For this review, take the finished solid that the model builds, in its own axes (mm). Round coordinates to 2 decimals unless told otherwise and drop trailing zeros. Write each loop counter-clockwise with the first axis right and the second up, starting at its lowest first coordinate (ties: lowest second). Pieces come first, ordered by that corner, then holes. Notation, with made-up numbers: (-37.75, -12) -> (-25.75, -12) arc R8 ccw to (-25.75, 3) -> close; hole circle Ø2 at (51, 53.25). An arc over 180 degrees is marked (long way). Answer as CSV lines item,"result". Start each with the question number.
Item 1: For pin 1 Ø8 at (x, y) = (50, 0) entering from +Z, flat-tipped, find the tip position at first contact; note if it passes through.
Item 2: Take a section at A-A on x = 50. Give the boundary of the cut face in (y, z), then the cut area to 3 significant figures.
Item 3: Take a section at B-B on y = 0. Give the boundary of the cut face in (x, z), then the cut area to 3 significant figures.
Item 4: Take a section at D-D on y = 4.75. Give the boundary of the cut face in (x, z), then the cut area to 3 significant figures.
Item 5: Take a section at C-C on z = 0.45. Give the boundary of the cut face in (x, y).
Item 6: Wall thickness on probe 1 along Y at (x, z) = (-50, -0.65); probe 2 along X at (y, z) = (3.5, 0.75); probe 3 along X at (y, z) = (-2, -1): over which ranges is each line inside the solid? List them lowest first. Write a range as from..to.
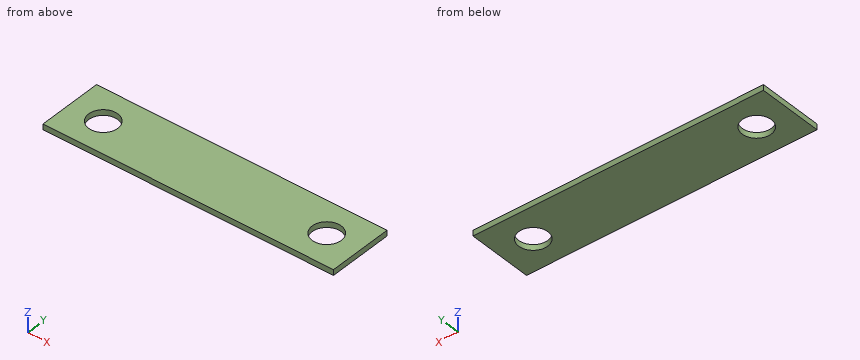
Autodesk Inventor part; units mm, degrees
ref_plane "YZ Plane" through (0, 0, 0) normal (1, 0, 0) x (0, 1, 0)
ref_plane "XZ Plane" through (0, 0, 0) normal (0, 1, 0) x (-1, 0, 0)
ref_plane "XY Plane" through (0, 0, 0) normal (0, 0, 1) x (1, 0, 0)
sketch "草圖1" plane through (0, 0, 0) normal (0, 0, 1) x (1, 0, 0)
  line L0 (0, 0) -> (-50, 0) construction
  line L1 (0, 0) -> (0, 45.4619) construction
  line L2 (-65, -14.5) -> (65, -14.5)
  line L3 (65, -14.5) -> (65, 14.5)
  line L4 (65, 14.5) -> (-65, 14.5)
  line L5 (-65, 14.5) -> (-65, -14.5)
  line L6 (-65, -14.5) -> (65, 14.5) construction
  line L7 (65, -14.5) -> (-65, 14.5) construction
  circle A0 centre (-50, 0) radius 6.5
  circle A1 centre (50, 0) radius 6.5
  dimension "d0" = 29
  dimension "d1" = 130
  dimension "d5" = 13
  dimension "d6" = 100
extrude "擠出1" add sketch "草圖1" along normal mid plane 2.5
properties part number "0 零件" material "橡膠"
Output values:
1,pin 1,"passes through"
2,outline,"(-14.5, -1.25) -> (-6.5, -1.25) -> (-6.5, 1.25) -> (-14.5, 1.25) -> close; (6.5, -1.25) -> (14.5, -1.25) -> (14.5, 1.25) -> (6.5, 1.25) -> close"
2,area,"40.0 mm^2"
3,outline,"(-65, -1.25) -> (-56.5, -1.25) -> (-56.5, 1.25) -> (-65, 1.25) -> close; (-43.5, -1.25) -> (43.5, -1.25) -> (43.5, 1.25) -> (-43.5, 1.25) -> close; (56.5, -1.25) -> (65, -1.25) -> (65, 1.25) -> (56.5, 1.25) -> close"
3,area,"260 mm^2"
4,outline,"(-65, -1.25) -> (-54.44, -1.25) -> (-54.44, 1.25) -> (-65, 1.25) -> close; (-45.56, -1.25) -> (45.56, -1.25) -> (45.56, 1.25) -> (-45.56, 1.25) -> close; (54.44, -1.25) -> (65, -1.25) -> (65, 1.25) -> (54.44, 1.25) -> close"
4,area,"281 mm^2"
5,outline,"(-65, -14.5) -> (65, -14.5) -> (65, 14.5) -> (-65, 14.5) -> close; hole circle Ø13 at (-50, 0); hole circle Ø13 at (50, 0)"
6,probe 1,"y = -14.5..-6.5, 6.5..14.5"
6,probe 2,"x = -65..-55.48, -44.52..44.52, 55.48..65"
6,probe 3,"x = -65..-56.18, -43.82..43.82, 56.18..65"
